Verification items for this drawing (mm, ordinates from the low corner). A direction names the side the tool comes from. Coordinates: 2 decimals unless noted, no trailing zeros. Write each loop counter-clockwise with the first axis right and the second up, starting at its lowest first coordinate (ties: lowest second). Pieces come first, ordered by that corner, then holes.
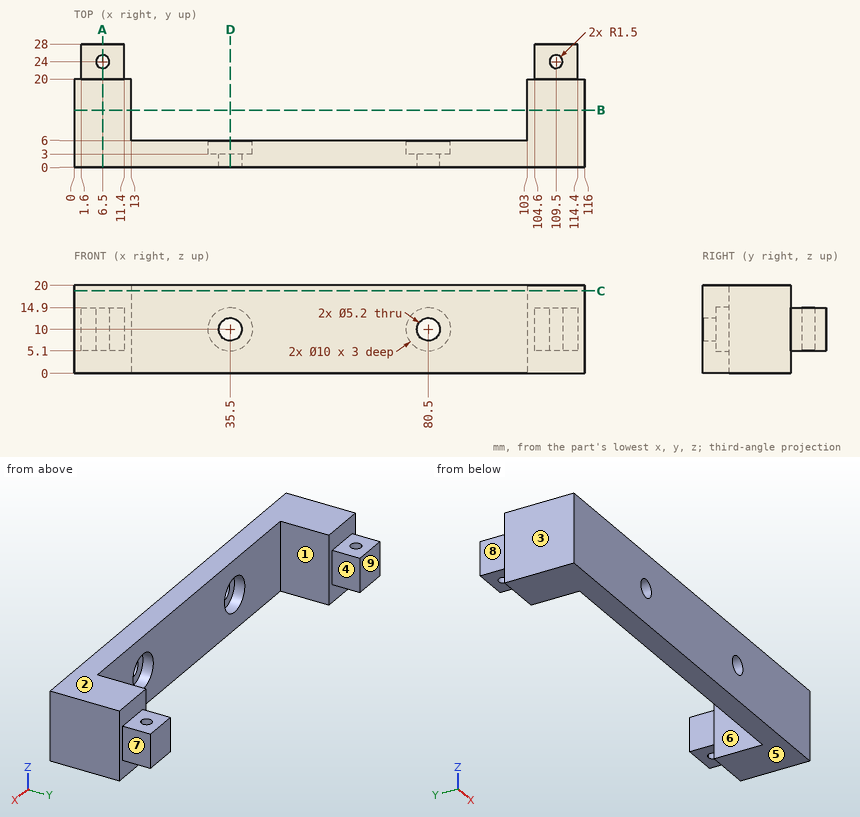
1. Gauge pin test, flat ends, axial feed: pin 1 Ø2 at (x, z) = (45, 6.5) entering from +Y; pin 2 Ø8 at (x, z) = (35.5, 10) entering from +Y; pin 3 Ø2.5 at (y, z) = (22.5, 10) entering from -X; pin 4 Ø3 at (x, z) = (80.5, 10) entering from +Y. Record the tip position at first contact, or that the pin passes through.
Computed values:
pin 1: stops at y = 6
pin 2: stops at y = 3
pin 3: stops at x = 1.6
pin 4: passes through
2. Sectioned sample at C-C, the plane z = 18.75. Record the boundary of the cut face in (x, y), and give its area (3 significant figures).
Computed values:
outline: (0, 0) - (116, 0) - (116, 20) - (103, 20) - (103, 6) - (13, 6) - (13, 20) - (0, 20) - close
area: 1,060 mm2
3. Draft check along X on the marked faces 1, 2, 3 and 4. Enter one of: released by +X, released by -X, zero draft, split by the parting line, or undercut.
Computed values:
face 1: undercut
face 2: zero draft
face 3: released by -X
face 4: undercut
4. Thickness scan on line 1 along X through (y, z) = (19.75, 11.25); line 2 along X through (y, z) = (4.95, 10); line 3 along Z through (x, y) = (80.5, 2.35). Record the ranges inside material, lowest first.
Computed values:
line 1: x = 0 to 13, 103 to 116
line 2: x = 0 to 30.5, 40.5 to 75.5, 85.5 to 116
line 3: z = 0 to 7.4, 12.6 to 20
5. Access from +Z, -Z, +X, -X, +Y, -Y to the whole of each face (thin tool, end or side, straight path). Record for the marked faces 5, 6, 7, 8 and 9.
Computed values:
face 5: -Z, +X, -X, +Y, -Y
face 6: +Z, -Z, +Y
face 7: +Z, -Z, +X, +Y
face 8: +Z, -Z, -X, +Y
face 9: +Z, -Z, +X, -X, +Y
6. Sectioned sample at A-A, the plane x = 6.5. Record the boundary of the cut face in (y, z), and give its area (3 significant figures).
Computed values:
outline: (0, 0) - (20, 0) - (20, 5.1) - (22.5, 5.1) - (22.5, 14.9) - (20, 14.9) - (20, 20) - (0, 20) - close; (25.5, 5.1) - (28, 5.1) - (28, 14.9) - (25.5, 14.9) - close
area: 449 mm2
7. Sectioned sample at B-B, the plane y = 13. Record the boundary of the cut face in (x, z).
Computed values:
outline: (0, 0) - (13, 0) - (13, 20) - (0, 20) - close; (103, 0) - (116, 0) - (116, 20) - (103, 20) - close
8. Sectioned sample at D-D, the plane x = 35.5. Record the boundary of the cut face in (y, z), and give its area (3 significant figures).
Computed values:
outline: (0, 0) - (6, 0) - (6, 5) - (3, 5) - (3, 7.4) - (0, 7.4) - close; (0, 12.6) - (3, 12.6) - (3, 15) - (6, 15) - (6, 20) - (0, 20) - close
area: 74.4 mm2
